Here's how the part is built. I have some questions about the finished solid (model axes, mm). Face numbers are marked on the shaded views. Round coordinates to 2 decimals unless told otherwise and drop trailing zeros. Write each loop counter-clockwise with the first axis right and the second up, starting at its lowest first coordinate (ties: lowest second). Pieces come first, ordered by that corner, then holes. Notation, with made-up numbers: (18, 78.5) - (31, 78.5) arc R20 ccw to (31, 106.5) - close; hole circle Ø2 at (1, -20). An arc over 180 degrees is marked (long way). Return JSON: item names as keys, results as strings. Group by question number.
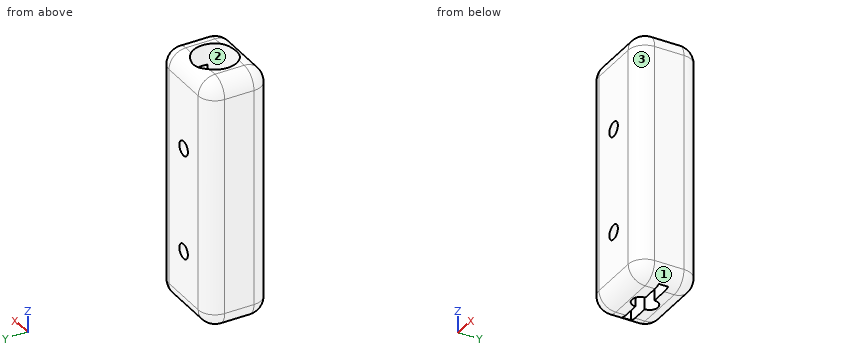
```python
from build123d import *

# Parameters (mm, degrees)
SKETCH1_W           = 20
SKETCH1_H           = 15
BOSS_EXTRUDE1_DEPTH = 60
SKETCH2_R           = 5.15
CUT_EXTRUDE1_DEPTH  = 55
SKETCH3_W           = 15.2
SKETCH3_H           = 2.2
CUT_EXTRUDE2_DEPTH  = 55
SKETCH4_R           = 1.75
CUT_EXTRUDE3_DEPTH  = 66
FILLET1_R           = 4
FILLET3_R           = 4
CUT_EXTRUDE4_REACH  = 67


with BuildPart() as part:
    # Sketch1 → Boss-Extrude1 (new body)
    with BuildSketch(Plane.XY):
        with Locations((10, 7.5)):
            Rectangle(SKETCH1_W, SKETCH1_H)
    extrude(amount=BOSS_EXTRUDE1_DEPTH)

    # Sketch2 → Cut-Extrude1 (cut)
    with BuildSketch(Plane.XY.offset(60)):
        with Locations((10, 7.5)):
            Circle(SKETCH2_R)
    extrude(amount=-CUT_EXTRUDE1_DEPTH, mode=Mode.SUBTRACT)

    # Sketch3 → Cut-Extrude2 (cut)
    with BuildSketch(Plane(origin=(0, 0, 0), x_dir=(-1, 0, 0), z_dir=(0, 0, -1))):
        with Locations((-10, 7.5)):
            Rectangle(SKETCH3_W, SKETCH3_H)
    extrude(amount=-CUT_EXTRUDE2_DEPTH, mode=Mode.SUBTRACT)

    # Sketch4 → Cut-Extrude3 (cut, through all)
    with BuildSketch(Plane(origin=(0, 15, 0), x_dir=(1, 0, 0), z_dir=(0, 1, 0))):
        with Locations(Location((10, -15, 0), (0, 0, 270))):
            Circle(SKETCH4_R)
        with Locations(Location((10, -40, 0), (0, 0, 270))):
            Circle(SKETCH4_R)
    extrude(amount=-CUT_EXTRUDE3_DEPTH, mode=Mode.SUBTRACT)

    # Fillet1
    # the kernel refuses this fillet: 4 mm, written as the material it takes off along each edge
    with BuildSketch(Plane(origin=(0, 15, -10), x_dir=(0, -1, 0), z_dir=(0, 0, 1)), Plane(origin=(0, 0, -10), x_dir=(1, 0, 0), z_dir=(0, 0, 1))) as fillet1_piece_1:
        with BuildLine():
            CenterArc((FILLET1_R, FILLET1_R), FILLET1_R, 180, 90)
            Line((0, FILLET1_R), (0, 0))
            Line((0, 0), (FILLET1_R, 0))
        make_face()
    extrude(amount=80, mode=Mode.SUBTRACT)
    with BuildSketch(Plane(origin=(0, 25, 60), x_dir=(0, 0, -1), z_dir=(0, -1, 0)), Plane(origin=(20, -10, 0), x_dir=(-1, 0, 0), z_dir=(0, 1, 0))) as fillet1_piece_2:
        with BuildLine():
            CenterArc((FILLET1_R, FILLET1_R), FILLET1_R, 180, 90)
            Line((0, FILLET1_R), (0, 0))
            Line((0, 0), (FILLET1_R, 0))
        make_face()
    extrude(amount=35, mode=Mode.SUBTRACT)
    with BuildSketch(Plane(origin=(0, 25, 0), x_dir=(0, 0, 1), z_dir=(0, -1, 0)), Plane(origin=(20, -10, 60), x_dir=(-1, 0, 0), z_dir=(0, 1, 0))) as fillet1_piece_3:
        with BuildLine():
            CenterArc((FILLET1_R, -FILLET1_R), FILLET1_R, 90, 90)
            Line((0, -FILLET1_R), (0, 0))
            Line((0, 0), (FILLET1_R, 0))
        make_face()
    extrude(amount=35, mode=Mode.SUBTRACT)
    with BuildSketch(Plane(origin=(20, 0, -10), x_dir=(-1, 0, 0), z_dir=(0, 0, 1)), Plane(origin=(20, 15, -10), x_dir=(0, -1, 0), z_dir=(0, 0, 1))) as fillet1_piece_4:
        with BuildLine():
            CenterArc((FILLET1_R, -FILLET1_R), FILLET1_R, 90, 90)
            Line((0, -FILLET1_R), (0, 0))
            Line((0, 0), (FILLET1_R, 0))
        make_face()
    extrude(amount=80, mode=Mode.SUBTRACT)

    # Fillet3
    # the kernel refuses this fillet: 4 mm, written as the material it takes off along each edge
    with BuildSketch(Plane(origin=(4, 4, 56), x_dir=(0, 0, 1), z_dir=(0, -1, 0))) as fillet3_piece_1_section:
        Polygon((0, 0), (FILLET3_R, 0), (FILLET3_R, FILLET3_R), (0, FILLET3_R), align=None)
    fillet3_piece_1 = extrude(amount=FILLET3_R, mode=Mode.PRIVATE)
    fillet3_piece_1 = fillet3_piece_1 - Plane(origin=(4, 4, 56), x_dir=(0.7071067811865475, 0, -0.7071067811865475), z_dir=(0, -1, 0)) * Sphere(FILLET3_R, mode=Mode.PRIVATE)
    add(fillet3_piece_1, mode=Mode.SUBTRACT)
    with BuildSketch(Plane(origin=(4, 4, 4), x_dir=(0, 0, -1), z_dir=(0, -1, 0))) as fillet3_piece_2_section:
        Polygon((0, 0), (FILLET3_R, 0), (FILLET3_R, -FILLET3_R), (0, -FILLET3_R), align=None)
    fillet3_piece_2 = extrude(amount=FILLET3_R, mode=Mode.PRIVATE)
    fillet3_piece_2 = fillet3_piece_2 - Plane(origin=(4, 4, 4), x_dir=(0.7071067811865475, 0, 0.7071067811865475), z_dir=(0, -1, 0)) * Sphere(FILLET3_R, mode=Mode.PRIVATE)
    add(fillet3_piece_2, mode=Mode.SUBTRACT)
    with BuildSketch(Plane(origin=(4, 11, 56), x_dir=(0, 1, 0), z_dir=(0, 0, 1))) as fillet3_piece_3_section:
        Polygon((0, 0), (FILLET3_R, 0), (FILLET3_R, FILLET3_R), (0, FILLET3_R), align=None)
    fillet3_piece_3 = extrude(amount=FILLET3_R, mode=Mode.PRIVATE)
    fillet3_piece_3 = fillet3_piece_3 - Plane(origin=(4, 11, 56), x_dir=(0.7071067811865475, -0.7071067811865475, 0), z_dir=(0, 0, 1)) * Sphere(FILLET3_R, mode=Mode.PRIVATE)
    add(fillet3_piece_3, mode=Mode.SUBTRACT)
    with BuildSketch(Plane(origin=(4, 11, 4), x_dir=(0, 0, -1), z_dir=(0, 1, 0))) as fillet3_piece_4_section:
        Polygon((0, 0), (FILLET3_R, 0), (FILLET3_R, FILLET3_R), (0, FILLET3_R), align=None)
    fillet3_piece_4 = extrude(amount=FILLET3_R, mode=Mode.PRIVATE)
    fillet3_piece_4 = fillet3_piece_4 - Plane(origin=(4, 11, 4), x_dir=(0.7071067811865475, 0, 0.7071067811865475), z_dir=(0, 1, 0)) * Sphere(FILLET3_R, mode=Mode.PRIVATE)
    add(fillet3_piece_4, mode=Mode.SUBTRACT)
    with BuildSketch(Plane(origin=(16, 11, 56), x_dir=(0, 1, 0), z_dir=(0, 0, 1))) as fillet3_piece_5_section:
        Polygon((0, 0), (FILLET3_R, 0), (FILLET3_R, -FILLET3_R), (0, -FILLET3_R), align=None)
    fillet3_piece_5 = extrude(amount=FILLET3_R, mode=Mode.PRIVATE)
    fillet3_piece_5 = fillet3_piece_5 - Plane(origin=(16, 11, 56), x_dir=(-0.7071067811865475, -0.7071067811865475, 0), z_dir=(0, 0, 1)) * Sphere(FILLET3_R, mode=Mode.PRIVATE)
    add(fillet3_piece_5, mode=Mode.SUBTRACT)
    with BuildSketch(Plane(origin=(16, 11, 4), x_dir=(0, 0, -1), z_dir=(0, 1, 0))) as fillet3_piece_6_section:
        Polygon((0, 0), (FILLET3_R, 0), (FILLET3_R, -FILLET3_R), (0, -FILLET3_R), align=None)
    fillet3_piece_6 = extrude(amount=FILLET3_R, mode=Mode.PRIVATE)
    fillet3_piece_6 = fillet3_piece_6 - Plane(origin=(16, 11, 4), x_dir=(-0.7071067811865475, 0, 0.7071067811865475), z_dir=(0, 1, 0)) * Sphere(FILLET3_R, mode=Mode.PRIVATE)
    add(fillet3_piece_6, mode=Mode.SUBTRACT)
    with BuildSketch(Plane(origin=(16, 4, 56), x_dir=(0, 0, 1), z_dir=(0, -1, 0))) as fillet3_piece_7_section:
        Polygon((0, 0), (FILLET3_R, 0), (FILLET3_R, -FILLET3_R), (0, -FILLET3_R), align=None)
    fillet3_piece_7 = extrude(amount=FILLET3_R, mode=Mode.PRIVATE)
    fillet3_piece_7 = fillet3_piece_7 - Plane(origin=(16, 4, 56), x_dir=(-0.7071067811865475, 0, -0.7071067811865475), z_dir=(0, -1, 0)) * Sphere(FILLET3_R, mode=Mode.PRIVATE)
    add(fillet3_piece_7, mode=Mode.SUBTRACT)
    with BuildSketch(Plane(origin=(16, 4, 4), x_dir=(0, 0, -1), z_dir=(0, -1, 0))) as fillet3_piece_8_section:
        Polygon((0, 0), (FILLET3_R, 0), (FILLET3_R, FILLET3_R), (0, FILLET3_R), align=None)
    fillet3_piece_8 = extrude(amount=FILLET3_R, mode=Mode.PRIVATE)
    fillet3_piece_8 = fillet3_piece_8 - Plane(origin=(16, 4, 4), x_dir=(-0.7071067811865475, 0, 0.7071067811865475), z_dir=(0, -1, 0)) * Sphere(FILLET3_R, mode=Mode.PRIVATE)
    add(fillet3_piece_8, mode=Mode.SUBTRACT)
    with BuildSketch(Plane(origin=(16, 15, 0), x_dir=(0, 0, 1), z_dir=(-1, 0, 0)), Plane(origin=(16, 15, 60), x_dir=(0, -1, 0), z_dir=(-1, 0, 0)), Plane(origin=(4, 0, 0), x_dir=(0, 0, 1), z_dir=(1, 0, 0))) as fillet3_piece_9:
        with BuildLine():
            CenterArc((FILLET3_R, -FILLET3_R), FILLET3_R, 90, 90)
            Line((0, -FILLET3_R), (0, 0))
            Line((0, 0), (FILLET3_R, 0))
        make_face()
    extrude(amount=12, mode=Mode.SUBTRACT)
    with BuildSketch(Plane(origin=(4, 0, 60), x_dir=(0, 0, -1), z_dir=(1, 0, 0))) as fillet3_piece_10:
        with BuildLine():
            CenterArc((FILLET3_R, FILLET3_R), FILLET3_R, 180, 90)
            Line((0, FILLET3_R), (0, 0))
            Line((0, 0), (FILLET3_R, 0))
        make_face()
    extrude(amount=12, mode=Mode.SUBTRACT)

    # Sketch5 → Cut-Extrude4 (cut, up to next)
    with BuildSketch(Plane(origin=(0, 0, 0), x_dir=(-1, 0, 0), z_dir=(0, 0, -1)), mode=Mode.PRIVATE) as cut_extrude4_sk1:
        with BuildLine():
            Line((-12, 8.6), (-8, 8.6))
            ThreePointArc((-8, 8.6), (-10, 10.6), (-12, 8.6))
        make_face()
    cut_extrude4_tool1 = extrude(cut_extrude4_sk1.sketch, amount=-CUT_EXTRUDE4_REACH, mode=Mode.PRIVATE) & part.part
    # Sketch5 → Cut-Extrude4 (cut, up to next)
    with BuildSketch(Plane(origin=(0, 0, 0), x_dir=(-1, 0, 0), z_dir=(0, 0, -1)), mode=Mode.PRIVATE) as cut_extrude4_sk2:
        with BuildLine():
            Line((-12.002485504, 6.4), (-7.997514496, 6.4))
            ThreePointArc((-7.997514496, 6.4), (-10, 4.397514496), (-12.002485504, 6.4))
        make_face()
    cut_extrude4_tool2 = extrude(cut_extrude4_sk2.sketch, amount=-CUT_EXTRUDE4_REACH, mode=Mode.PRIVATE) & part.part
    add(cut_extrude4_tool1.solids().sort_by_distance((10, 9.448826, 0))[0], mode=Mode.SUBTRACT)
    add(cut_extrude4_tool2.solids().sort_by_distance((10, 5.550119, 0))[0], mode=Mode.SUBTRACT)


solid = part.part
```
1) Imagine slicing it at A-A (z = 15). Please give me the cut outline in (x, y).
2) I need wall thicknesses on line 1 along Z through (x, y) = (10, 1.8); line 2 along X through (y, z) = (8.75, 38.5); line 3 along X through (y, z) = (8, 38). Which ranges of each line are inside material? Lowest first, please.
3) Imagine slicing it at B-B (y = 7.5). Please give me the cut outline in (x, z).
4) Will these pins go through, and if not, where does the flat tip stop? pin 1 Ø1.1 at (x, y) = (17, 7.5) entering from -Z; pin 2 Ø4.5 at (x, y) = (10.5, 10) entering from +Z; pin 3 Ø2 at (y, z) = (12.5, 40) entering from +X.
5) If we mould it in two halves opening along Y, with no side actions, what happens to the marked faces 1, 2 and 3? For each: released by +Y, released by -Y, zero draft, split by the parting line, or undercut.
6) Imagine slicing it at D-D (x = 10). Give the number of separate pieces and of enclosed holes in the cut face, plus the area to 3 significant figures.
7) Imagine slicing it at C-C (z = 48.5). Please give me the cut outline in (x, y), plus the area to 3 significant figures.
Results found:
{
 "1": {"outline": "(0, 4) arc R4 ccw to (4, 0) - (8.25, 0) - (8.25, 2.66) arc R5.15 cw to (4.97, 6.4) - (2.4, 6.4) - (2.4, 8.6) - (4.97, 8.6) arc R5.15 cw to (8.25, 12.34) - (8.25, 15) - (4, 15) arc R4 ccw to (0, 11) - close; (11.75, 0) - (16, 0) arc R4 ccw to (20, 4) - (20, 11) arc R4 ccw to (16, 15) - (11.75, 15) - (11.75, 12.34) arc R5.15 cw to (15.03, 8.6) - (17.6, 8.6) - (17.6, 6.4) - (15.03, 6.4) arc R5.15 cw to (11.75, 2.66) - close"},
 "2": {"line 1": "z = 0.66 to 13.25, 16.75 to 38.25, 41.75 to 59.34", "line 2": "x = 0 to 5, 15 to 20", "line 3": "x = 0 to 2.4, 17.6 to 20"},
 "3": {"outline": "(0, 4) arc R4 ccw to (2.4, 0.33) - (2.4, 55) - (4.85, 55) - (4.85, 60) - (4, 60) arc R4 ccw to (0, 56) - close; (15.15, 55) - (17.6, 55) - (17.6, 0.33) arc R4 ccw to (20, 4) - (20, 56) arc R4 ccw to (16, 60) - (15.15, 60) - close"},
 "4": {"pin 1": "stops at z = 55", "pin 2": "stops at z = 5", "pin 3": "stops at x = 19.97"},
 "5": {"face 1": "zero draft", "face 2": "undercut", "face 3": "released by -Y"},
 "6": {"separate pieces": "6", "enclosed holes": "0", "area": "256 mm²"},
 "7": {"outline": "(0, 4) arc R4 ccw to (4, 0) - (16, 0) arc R4 ccw to (20, 4) - (20, 11) arc R4 ccw to (16, 15) - (4, 15) arc R4 ccw to (0, 11) - close; hole (2.4, 6.4) - (4.97, 6.4) arc R5.15 ccw to (15.03, 6.4) - (17.6, 6.4) - (17.6, 8.6) - (15.03, 8.6) arc R5.15 ccw to (4.97, 8.6) - (2.4, 8.6) - close", "area": "192 mm²"}
}
